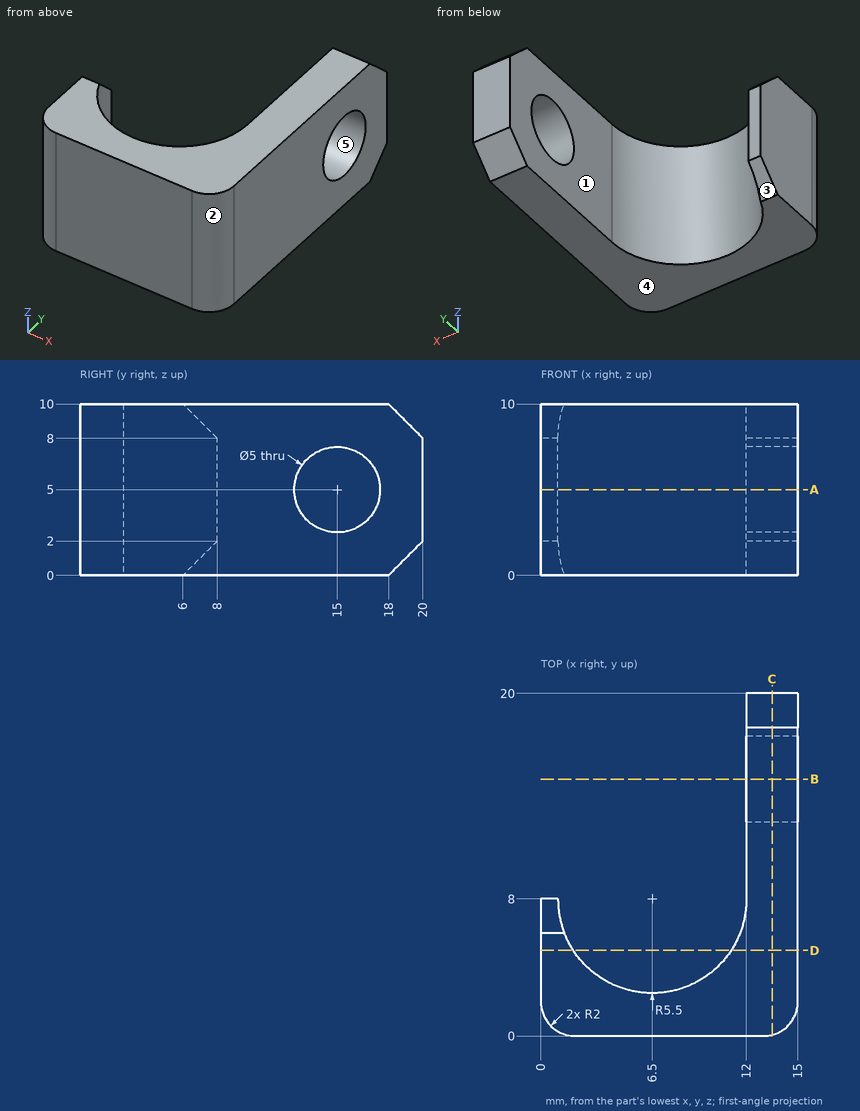
The drawing under review shows one solid part. Ordinate dimensions are in mm from its lowest x, y, z. A direction names the side the tool comes from. Give positions to 0.01 mm unless a question says otherwise; leave off trailing zeros. Write each loop counter-clockwise with the first axis right and the second up, starting at its lowest first coordinate (ties: lowest second). Pieces come first, ordered by that corner, then holes. Notation, with made-up numbers: (-4, 80) -> (37, 80) arc R24 ccw to (37, 100) -> close; hole circle Ø1 at (52, 87.25). An arc over 180 degrees is marked (long way). Put each result on its own line as item: value.
(1) The part is to be moulded in two halves that separate along Y. For the marked faces 3, 4 and 5, say which applies: pulls with the +Y half, pulls with the -Y half, needs draft (parallel to the pull), parting line crosses it, or undercut.
Results are:
face 3: pulls with the +Y half
face 4: needs draft
face 5: undercut
(2) To check wall thickness, follow probe 1 along Z at (x, y) = (13.35, 15); probe 2 along X at (y, z) = (13, 7.75); probe 3 along Y at (x, z) = (13.5, 6.5). State the ranges of each line that lie inside material, in increasing order. Write a range as from..to.
Results are:
probe 1: 0..2.5, 7.5..10
probe 2: 12..15
probe 3: 0.06..13, 17..20
(3) We need section D-D, the plane y = 5. Give the boundary of the cut face in (x, z).
Results are:
outline: (0, 0) -> (1.89, 0) -> (1.89, 10) -> (0, 10) -> close; (11.11, 0) -> (15, 0) -> (15, 10) -> (11.11, 10) -> close
(4) For pin 1 Ø1.1 at (x, z) = (0.5, 5) entering from +Y; pin 2 Ø2 at (x, z) = (5, 7.5) entering from +Y; pin 3 Ø1.5 at (x, z) = (8, 7.5) entering from +Y, all flat-tipped, find the tip position at first contact; note any pin that passes through.
Results are:
pin 1: y = 8
pin 2: y = 3.1
pin 3: y = 2.98
(5) We need section C-C, the plane x = 13.5. Give the boundary of the cut face in (y, z), and give its area (3 significant figures).
Results are:
outline: (0.06, 0) -> (18, 0) -> (20, 2) -> (20, 8) -> (18, 10) -> (0.06, 10) -> close; hole circle Ø5 at (15, 5)
area: 176 mm²
(6) Tool access review of the marked faces 1 and 2: name each direction out of +Z, -Z, +X, -X, +Y, -Y from which nothing blocks a thin tool from reaching the whole face with its end or side.
Results are:
face 1: +Z, -Z, -X, +Y
face 2: +Z, -Z, +X, -Y
(7) We need section B-B, the plane y = 15. Give the boundary of the cut face in (x, z).
Results are:
outline: (12, 0) -> (15, 0) -> (15, 2.5) -> (12, 2.5) -> close; (12, 7.5) -> (15, 7.5) -> (15, 10) -> (12, 10) -> close
(8) We need section A-A, the plane z = 5. Give the boundary of the cut face in (x, y).
Results are:
outline: (0, 2) arc R2 ccw to (2, 0) -> (13, 0) arc R2 ccw to (15, 2) -> (15, 12.5) -> (12, 12.5) -> (12, 8) arc R5.5 cw to (1, 8) -> (0, 8) -> close; (12, 17.5) -> (15, 17.5) -> (15, 20) -> (12, 20) -> close
